from build123d import *

# Parameters (mm, degrees)
ESQUISSE1_R             = 38
ESQUISSE1_R_2           = 35
BOSS_EXTRU_1_DEPTH      = 10
BOSS_EXTRU_2_START      = 3
ESQUISSE2_R             = 38
BOSS_EXTRU_2_DEPTH      = 3
BOSS_EXTRU_3_DEPTH      = 3
ENL_V_MAT_EXTRU_1_DEPTH = 99.203869578
BOSS_EXTRU_4_DEPTH      = 6
CONG_1_R                = 10
CONG_3_R                = 1
CONG_4_R                = 1.5


with BuildPart() as part:
    # Esquisse1 → Boss.-Extru.1 (new body)
    with BuildSketch(Plane.XY):
        Circle(ESQUISSE1_R)
        Circle(ESQUISSE1_R_2, mode=Mode.SUBTRACT)
    extrude(amount=BOSS_EXTRU_1_DEPTH)

    # Esquisse2 → Boss.-Extru.2 (add)
    with BuildSketch(Plane(origin=(0, 0, 0), x_dir=(-1, 0, 0), z_dir=(0, 0, -1)).offset(BOSS_EXTRU_2_START)):
        Circle(ESQUISSE2_R)
    extrude(amount=-BOSS_EXTRU_2_DEPTH)

    # Esquisse3 → Boss.-Extru.3 (add)
    with BuildSketch(Plane.XY):
        Polygon((-5, -90), (5, -90), (25.656199867, -28.0314004), (-25.656199867, -28.0314004), align=None)
    extrude(amount=-BOSS_EXTRU_3_DEPTH)

    # Esquisse4 → Enlèv. mat.-Extru.1 (cut, through all)
    with BuildSketch(Plane.XY):
        Polygon((-19.037588305, -32.887235085), (-17.534620807, -30.29087442), (17.534620807, -30.29087442), (19.037588305, -32.887235085), (0, -90), align=None)
    extrude(amount=ENL_V_MAT_EXTRU_1_DEPTH, mode=Mode.SUBTRACT)

    # Esquisse5 → Boss.-Extru.4 (add)
    with BuildSketch(Plane.XY):
        Polygon((-5, -90), (-25.656199867, -28.0314004), (-17.534620807, -30.29087442), (-2.5, -90), align=None)
        Polygon((2.5, -90), (5, -90), (25.656199867, -28.0314004), (17.534620807, -30.29087442), align=None)
    extrude(amount=BOSS_EXTRU_4_DEPTH)

    # Congé1
    # the kernel refuses this fillet: 10 mm, written as the material it adds along each edge
    with BuildSketch(Plane(origin=(25.656199867, -28.0314004, 6), x_dir=(0.7181222649547252, 0.6959169581036918, 0), z_dir=(0, 0, -1)), Plane(origin=(-25.656199867, -28.0314004, -3), x_dir=(-0.7181222649547252, 0.6959169581036918, 0), z_dir=(0, 0, 1))) as cong_1_piece_1:
        with BuildLine():
            CenterArc((2.451539853, 9.995936135), CONG_1_R, 242.53528085, 25.831208482)
            Line((-2.160483484, 1.122986189), (0, 0))
            ThreePointArc((0, 0), (1.08323854, 0.015442687), (2.16647708, 0))
        make_face()
    extrude(amount=9)
    # the kernel refuses this fillet: 10 mm, written as the material it takes off along each edge
    with BuildSketch(Plane(origin=(17.534620807, -30.29087442, 0), x_dir=(0.8396660922433514, 0.5431029861239759, 0), z_dir=(0, 0, 1))) as cong_1_2_piece_1:
        with BuildLine():
            CenterArc((3.949343583, -9.987807165), CONG_1_R, 92.829659135, 40.142072995)
            Line((-2.867030927, -2.670906281), (0, 0))
            ThreePointArc((0, 0), (1.727837818, -0.042674924), (3.455675635, 0))
        make_face()
    extrude(amount=15.795919653, mode=Mode.SUBTRACT)
    with BuildSketch(Plane(origin=(-17.534620807, -30.29087442, 0), x_dir=(-0.839666092243352, 0.5431029861239753, 0), z_dir=(0, 0, 1))) as cong_1_2_piece_2:
        with BuildLine():
            CenterArc((3.949343583, 9.987807165), CONG_1_R, 227.028267869, 40.142072995)
            Line((-2.867030927, 2.670906281), (0, 0))
            ThreePointArc((0, 0), (1.727837818, 0.042674924), (3.455675635, 0))
        make_face()
    extrude(amount=15.795919653, mode=Mode.SUBTRACT)

    # Congé3
    cong_3_edges = [part.edges().sort_by_distance(p)[0] for p in [
        (-2.5, -90, 3),
        (2.5, -90, 3),
    ]]
    fillet(cong_3_edges, radius=CONG_3_R)

    # Congé4
    cong_4_edges = [part.edges().sort_by_distance(p)[0] for p in [
        (-5, -90, 1.5),
        (5, -90, 1.5),
    ]]
    fillet(cong_4_edges, radius=CONG_4_R)


solid = part.part
Verification items for the finished model (mm, model axes). A direction names the side the tool comes from. Round coordinates to 2 decimals unless told otherwise and drop trailing zeros. Order: outer loops, then holes, each group sorted by start corner. A loop starts at its lowest first (then second) coordinate and runs counter-clockwise, first axis right, second up.
1. Go/stop test with flat-tipped pins: P1, Ø3, axis at x = 30, z = 0, coming from the +Y side; P2, Ø1, axis at y = -9.5, z = 2, coming from the -X side; P3, Ø3, axis at y = -28.5, z = 8, coming from the +X side. Record where each tip stops, or that it passes through.
Final values:
P1: stops at y = 25.13
P2: stops at x = -36.92
P3: stops at x = 26.74
2. Section check C-C on x = 0. Record the cut outline in (y, z), then the cut area to 3 significant figures.
Final values:
outline: (-90, -3) - (38, -3) - (38, 10) - (35, 10) - (35, 0) - (-90, 0) - close
area: 414 mm2
3. Section check A-A on z = 1.5. Record the cut outline in (x, y).
Final values:
outline: (-27.21, -26.52) arc R10 cw to (-24.89, -30.34) - (-5.34, -88.97) arc R1.5 ccw to (-3.92, -90) - (-3.78, -90) arc R1 ccw to (-2.81, -88.76) - (-16.58, -34.09) arc R10 ccw to (-20.44, -28.41) arc R35 cw (long way) to (20.44, -28.41) arc R10 ccw to (16.58, -34.09) - (2.81, -88.76) arc R1 ccw to (3.78, -90) - (3.92, -90) arc R1.5 ccw to (5.34, -88.97) - (24.89, -30.34) arc R10 cw to (27.21, -26.52) arc R38 ccw (long way) to start
4. Thickness scan on L1, parallel to X at y = 0, z = 6.25; L2, parallel to Z at x = -21.5, y = -5; L3, parallel to Y at x = 0, z = 4.5. Record the ranges inside material, lowest first.
Final values:
L1: x = -38 to -35, 35 to 38
L2: z = -3 to 0
L3: y = 35 to 38
5. Section check D-D on y = -74. Record the cut outline in (x, z), then the cut area to 3 significant figures.
Final values:
outline: (-10.33, -3) - (10.33, -3) - (10.33, 6) - (6.53, 6) - (6.53, 0) - (-6.53, 0) - (-6.53, 6) - (-10.33, 6) - close
area: 108 mm2
6. Access from +Z, -Z, +X, -X, +Y, -Y to the whole of each face (thin tool, end or side, straight path). Record for faces 1 (the flat face through (0, -13, 0)), 2 (the flat face through (0, -90, -1)).
Final values:
face 1: +Z
face 2: +Z, -Z, +X, -X, -Y
7. Section check B-B on y = 0. Record the cut outline in (x, z), then the cut area to 3 significant figures.
Final values:
outline: (-38, -3) - (38, -3) - (38, 10) - (35, 10) - (35, 0) - (-35, 0) - (-35, 10) - (-38, 10) - close
area: 288 mm2
